Can you work these out from the drawing? Everything is in mm from the part's minimum corner. A direction names the side the tool comes from. Give positions to 0.01 mm unless a question says otherwise; leave off trailing zeros. Order: outer loops, then holes, each group sorted by start corner. A loop starts at its lowest first (then second) coordinate and runs counter-clockwise, first axis right, second up. Notation, with made-up numbers: (71.5, -9) - (97.5, -9) arc R18 cw to (97.5, 12) - close; hole circle Ø7 at (53.5, 37.25). An arc over 180 degrees is marked (long way). Answer as a JSON object with one key per item and string values.
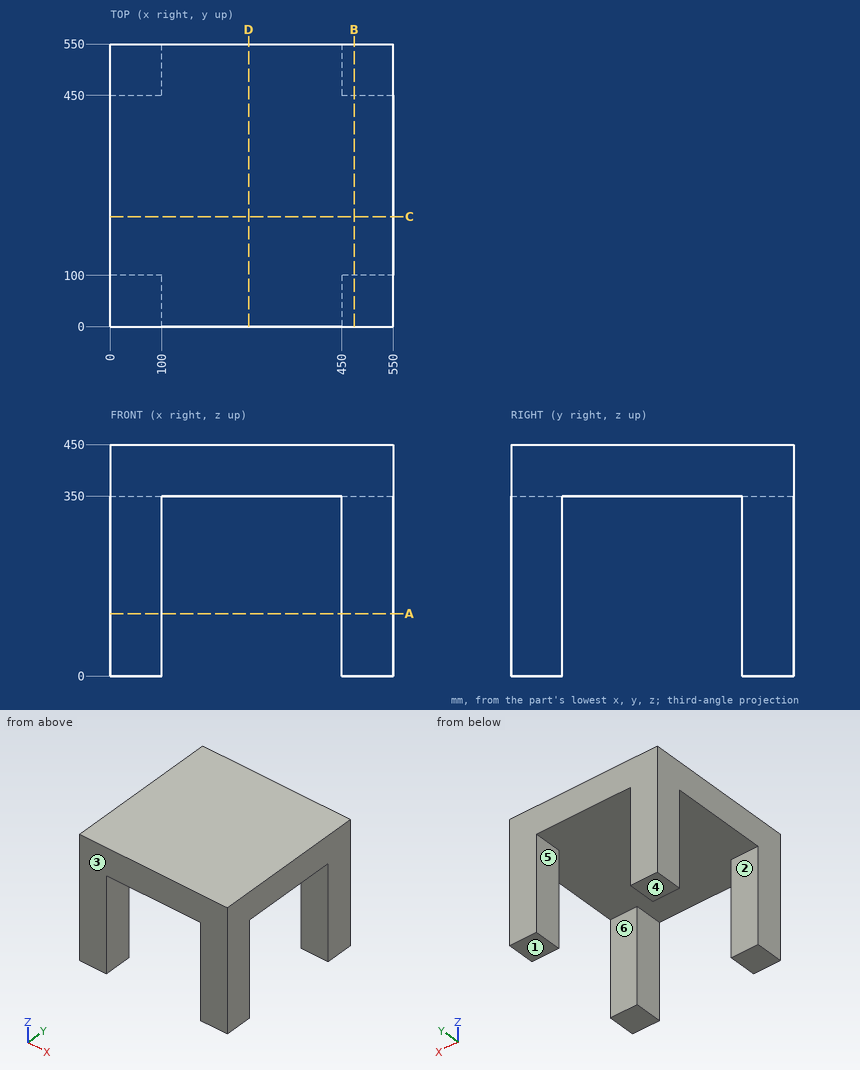
Q1. If we section it at A-A, the plane z = 121.5: Please give me the cut outline in (x, y), then the cut area to 3 significant figures.
Recorded:
{"outline": "(0, 0) - (100, 0) - (100, 100) - (0, 100) - close; (0, 450) - (100, 450) - (100, 550) - (0, 550) - close; (450, 0) - (550, 0) - (550, 100) - (450, 100) - close; (450, 450) - (550, 450) - (550, 550) - (450, 550) - close", "area": "40,000 mm^2"}
Q2. I need wall thicknesses on L1, parallel to X at y = 86, z = 52.5; L2, parallel to Z at x = 489.5, y = 404.5. Which ranges of each line are inside material? Lowest first, please.
Recorded:
{"L1": "x = 0 to 100, 450 to 550", "L2": "z = 350 to 450"}
Q3. If we section it at C-C, the plane y = 214: Please give me the cut outline in (x, z).
Recorded:
{"outline": "(0, 350) - (550, 350) - (550, 450) - (0, 450) - close"}
Q4. We'd pull the mould along Y, two halves only. Please class the marked faces 1, 2 and 3: released by +Y, released by -Y, zero draft, split by the parting line, or undercut.
Recorded:
{"face 1": "zero draft", "face 2": "undercut", "face 3": "released by -Y"}
Q5. Which directions (+Z, -Z, +X, -X, +Y, -Y) give clear straight access to the entire face, cutting with the end or side of a thin tool? Please do the marked faces 4, 5 and 6.
Recorded:
{"face 4": "-Z, +X, -X, +Y, -Y", "face 5": "-Z, +Y, -Y", "face 6": "-Z, +X, -X"}
Q6. I'm going to push a flat-ended pin straight in: pin 1 Ø1 at (x, y) = (135, 188) entering from -Z. Where does the tip first touch, or does it pass through?
Recorded:
{"pin 1": "stops at z = 350"}
Q7. If we section it at B-B, the plane x = 474.5: Please give me the cut outline in (y, z), then the cut area to 3 significant figures.
Recorded:
{"outline": "(0, 0) - (100, 0) - (100, 350) - (450, 350) - (450, 0) - (550, 0) - (550, 450) - (0, 450) - close", "area": "125,000 mm^2"}
